Autodesk Inventor part; units mm, degrees
ref_plane "YZ Plane" through (0, 0, 0) normal (1, 0, 0) x (0, 1, 0)
ref_plane "XZ Plane" through (0, 0, 0) normal (0, 1, 0) x (-1, 0, 0)
ref_plane "XY Plane" through (0, 0, 0) normal (0, 0, 1) x (1, 0, 0)
sketch "草圖1" plane through (0, 0, 0) normal (0, 0, 1) x (1, 0, 0)
  line L0 (0, 0) -> (-19.4073, 0) construction
  line L1 (0, 0) -> (0, 21.4127) construction
  line L2 (-3, 8.125) -> (-3, 3)
  arc A0 (-3, 3) -> (3, 3) centre (0, 3) ccw
  line L3 (3, 3) -> (3, 8.125)
  line L4 (1.25, 8.125) -> (1.25, 2)
  line L5 (-1.25, 2) -> (-1.25, 8.125)
  line L6 (-3, 9.712) -> (-3, 6.8385) construction
  line L7 (3, 9.712) -> (3, 6.8385) construction
  line L8 (-4.0339, 9) -> (4.2037, 9) construction
  line L9 (-1.25, 2) -> (1.25, 2)
  arc A1 (-1.25, 8.125) -> (-3, 8.125) centre (-2.125, 8.125) ccw
  arc A2 (3, 8.125) -> (1.25, 8.125) centre (2.125, 8.125) ccw
  dimension "d0" = 6
  dimension "d2" = 9
  dimension "d3" = 2
  dimension "d4" = 2.5
  dimension "d6" = 6
extrude "擠出1" add sketch "草圖1" along normal mid plane 130
properties part number "0 零件" material "橡膠"
Geometry check sheet. Reference: the model listing, model coordinates, mm. A direction names the side the tool comes from. Coordinates: 2 decimals unless noted, no trailing zeros. Loops run counter-clockwise (first coordinate to the right, second up) from the corner with the lowest first, then second, coordinate; pieces in that order, holes last.
Item 1: Go/stop test with flat-tipped pins: pin 1 Ø1.5 at (x, z) = (0.5, -45) entering from -Y; pin 2 Ø2 at (x, z) = (1, 18.5) entering from +Y; pin 3 Ø0.8 at (x, z) = (0.5, -16) entering from +Y. Record where each tip stops, or that it passes through.
Item 2: Sectioned sample at C-C, the plane x = 0. Record the boundary of the cut face in (y, z).
Item 3: Release check for a two-part mould opening along X. For faces 1 (the face through (-3, 6, -1)), 2 (the face through (3, 6, -1)), 3 (the face through (1.25, 5, -1)), 4 (the face through (-1.25, 5, -1)) record: released by +X, released by -X, zero draft, split by the parting line, or undercut.
Item 4: Access from +Z, -Z, +X, -X, +Y, -Y to the whole of each face (thin tool, end or side, straight path). Record for faces 5 (the face through (0, 2, -1)), 6 (the face through (0, 0, -1)).
Item 5: Thickness scan on line 1 (X direction, y = 4.25, z = 37.5); line 2 (Y direction, x = 0.85, z = 25.5); line 3 (Y direction, x = -1.75, z = -58). Record the ranges inside material, lowest first.
Item 6: Sectioned sample at B-B, the plane z = 34.5. Record the boundary of the cut face in (x, y) (3 decimals).
Item 7: Sectioned sample at A-A, the plane y = 4.75. Record the boundary of the cut face in (x, z), then the cut area to 3 significant figures.
Check result:
1. pin 1: stops at y = 0
1. pin 2: stops at y = 8.99
1. pin 3: stops at y = 2
2. outline: (0, -65) - (2, -65) - (2, 65) - (0, 65) - close
3. face 1: released by -X
3. face 2: released by +X
3. face 3: undercut
3. face 4: undercut
4. face 5: +Z, -Z, +Y
4. face 6: +Z, -Z, -Y
5. line 1: x = -3 to -1.25, 1.25 to 3
5. line 2: y = 0.12 to 2
5. line 3: y = 0.56 to 8.92
6. outline: (-3, 3) arc R3 ccw to (3, 3) - (3, 8.125) arc R0.875 ccw to (1.25, 8.125) - (1.25, 2) - (-1.25, 2) - (-1.25, 8.125) arc R0.875 ccw to (-3, 8.125) - close
7. outline: (-3, -65) - (-1.25, -65) - (-1.25, 65) - (-3, 65) - close; (1.25, -65) - (3, -65) - (3, 65) - (1.25, 65) - close
7. area: 455 mm2
